Work out the finished part from the listing and answer in its coordinate system (mm). Face numbers are marked on the shaded views. Give positions to 0.01 mm unless a question says otherwise; leave off trailing zeros. Loops run counter-clockwise (first coordinate to the right, second up) from the corner with the lowest first, then second, coordinate; pieces in that order, holes last. Notation, with made-up numbers: M 67.25,-4 L 89.25,-4 A29 ccw 89.25,17 Z; hole C 67.5,-25 d9. An arc over 180 degrees is marked long. Use a Markdown table: item, result.
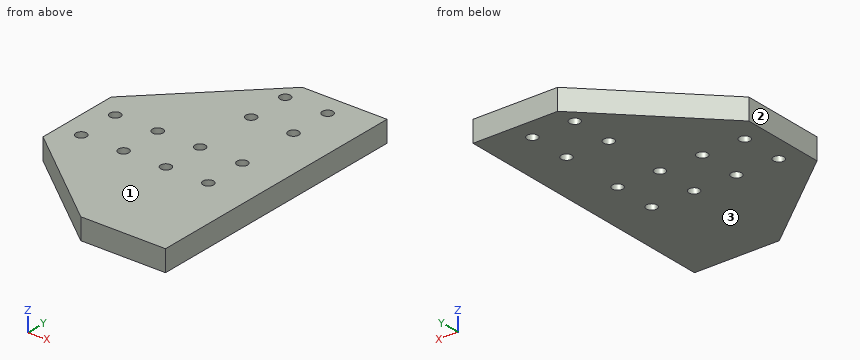
```python
from build123d import *

# Parameters (mm, degrees)
BOSS_EXTRUDE1_DEPTH = 10
SKETCH2_R           = 2.5
CUT_EXTRUDE1_DEPTH  = 10


with BuildPart() as part:
    # Sketch1 → Boss-Extrude1 (new body)
    with BuildSketch(Plane.XY):
        Polygon((0, 0), (40, 0), (40, 130), (0, 130), (-50, 80), (-50, 40), align=None)
    extrude(amount=BOSS_EXTRUDE1_DEPTH)

    # Sketch2 → Cut-Extrude1 (cut)
    with BuildSketch(Plane.XY.offset(10)):
        with Locations((0, 120)):
            Circle(SKETCH2_R)
        with Locations((20, 120)):
            Circle(SKETCH2_R)
        with Locations((0, 100)):
            Circle(SKETCH2_R)
        with Locations((20, 100)):
            Circle(SKETCH2_R)
        with Locations((-40, 70)):
            Circle(SKETCH2_R)
        with Locations((-20, 70)):
            Circle(SKETCH2_R)
        with Locations((-40, 50)):
            Circle(SKETCH2_R)
        with Locations((-20, 50)):
            Circle(SKETCH2_R)
        with Locations((0, 70)):
            Circle(SKETCH2_R)
        with Locations((20, 70)):
            Circle(SKETCH2_R)
        with Locations((0, 50)):
            Circle(SKETCH2_R)
        with Locations((20, 50)):
            Circle(SKETCH2_R)
    extrude(amount=-CUT_EXTRUDE1_DEPTH, mode=Mode.SUBTRACT)


solid = part.part
```
(1) Given P1, Ø3, axis at x = 20, y = 120, coming from the +Z side; P2, Ø6, axis at x = -12, z = 4, coming from the +Y side; P3, Ø2, axis at y = 103.5, z = 4, coming from the -X side; P4, Ø3, axis at x = -7, z = 6, coming from the -Y side, each flat-ended and moving along its own axis, determine where each tip first touches the part or whether it passes through.
Entries:
| item | result |
|---|---|
| P1 | passes through |
| P2 | stops at y = 121 |
| P3 | stops at x = -27.5 |
| P4 | stops at y = 4.4 |
(2) A cutting plane is placed at D-D (y = 100). Write down the section's boundary in (x, z).
Entries:
| item | result |
|---|---|
| outline | M -30,0 L -2.5,0 L -2.5,10 L -30,10 Z; M 2.5,0 L 17.5,0 L 17.5,10 L 2.5,10 Z; M 22.5,0 L 40,0 L 40,10 L 22.5,10 Z |
(3) A cutting plane is placed at A-A (y = 50). Write down the section's boundary in (x, z).
Entries:
| item | result |
|---|---|
| outline | M -50,0 L -42.5,0 L -42.5,10 L -50,10 Z; M -37.5,0 L -22.5,0 L -22.5,10 L -37.5,10 Z; M -17.5,0 L -2.5,0 L -2.5,10 L -17.5,10 Z; M 2.5,0 L 17.5,0 L 17.5,10 L 2.5,10 Z; M 22.5,0 L 40,0 L 40,10 L 22.5,10 Z |
(4) Consider probe 1 along Y at (x, z) = (20, 5.25); probe 2 along X at (y, z) = (98.5, 9.5); probe 3 along Y at (x, z) = (-40, 5.5). Determine where each line is inside the solid, lowest interval first. Write a range as [from, to].
Entries:
| item | result |
|---|---|
| probe 1 | y = [0, 47.5], [52.5, 67.5], [72.5, 97.5], [102.5, 117.5], [122.5, 130] |
| probe 2 | x = [-31.5, -2], [2, 18], [22, 40] |
| probe 3 | y = [32, 47.5], [52.5, 67.5], [72.5, 90] |
(5) The mould has two halves that part along Z. Classify the marked faces 1, 2 and 3: released by +Z, released by -Z, zero draft, split by the parting line, or undercut.
Entries:
| item | result |
|---|---|
| face 1 | released by +Z |
| face 2 | zero draft |
| face 3 | released by -Z |
(6) A cutting plane is placed at B-B (z = 6). Count the separate pieces of the cut face and the enclosed holes in it, and give its area (3 significant figures).
Entries:
| item | result |
|---|---|
| separate pieces | 1 |
| enclosed holes | 12 |
| area | 9,210 mm² |
(7) A cutting plane is placed at C-C (x = -40). Write down the section's boundary in (y, z).
Entries:
| item | result |
|---|---|
| outline | M 32,0 L 47.5,0 L 47.5,10 L 32,10 Z; M 52.5,0 L 67.5,0 L 67.5,10 L 52.5,10 Z; M 72.5,0 L 90,0 L 90,10 L 72.5,10 Z |
